Work out the finished part from the listing and answer in its coordinate system (mm). A direction names the side the tool comes from. Give positions to 0.01 mm unless a question says otherwise; leave off trailing zeros. Write each loop counter-clockwise with the first axis right and the second up, starting at its lowest first coordinate (ties: lowest second). Pieces come first, ordered by that corner, then holes. Notation, with made-up numbers: (85.25, 83.25) -> (136.25, 83.25) arc R22 ccw to (136.25, 109.25) -> close; hole circle Ø7 at (50, -21.75). An arc over 180 degrees is marked (long way). Use a Markdown table: item, result. Add a question column.
Q1. Section B-B, the plane z = -7.5 is taken. Give the vertices of the cut face in (x, y).
Q2. For faces 4 (the face through (-43, 10, -22.749)), 5 (the face through (-30.801, 10, -8)), 6 (the face through (-25, 9.25, 19)), 7 (the face through (-32, 14, 34.751)), determine the directions among +Z, -Z, +X, -X, +Y, -Y from which every point of the face is accessible in a straight line to the end or side of a thin tool.
Q3. Consider line 1 (X direction, y = 18.5, z = -2); line 2 (X direction, y = 7.5, z = -18); line 3 (X direction, y = 18.5, z = 15.5). Determine where each line is inside the solid, lowest interval first.
Q4. Section C-C, the plane x = -45 is taken. Give the vertices of the cut face in (y, z).
Q5. Section D-D, the plane z = 21 is taken. Give the vertices of the cut face in (x, y), plus the area to 3 significant figures.
Q6. For a pull along X with two mould halves and no side action, classify faces 1 (the face through (-26.999, 9.86, 9.807)), 2 (the face through (-51.47, 9.86, -29.92)), 3 (the face through (-25, 9.25, 41)) as pulls with the +X half, pulls with the -X half, needs draft (parallel to the pull), parting line crosses it, or undercut.
Q7. Section A-A, the plane y = 10 is taken. Give the vertices of the cut face in (x, z), plus the area to 3 significant figures.
Q8. Each of these flat-tipped pins is pushed along its axis until it touches: pin 1 Ø1 at (y, z) = (7, -4) entering from -X; pin 2 Ø1.6 at (x, y) = (-25, 10) entering from -Z; pin 3 Ø1.2 at (x, y) = (-27.5, 10) entering from -Z; pin 4 Ø2 at (x, z) = (-39.5, -7.5) entering from -Y. Where does it stop, or does it pass through?
from build123d import *

# Parameters (mm, degrees)
BOSS_EXTRUDE1_DEPTH = 20
SKETCH2_R           = 4
CUT_EXTRUDE2_DEPTH  = 8
SKETCH3_W           = 7.740011002
SKETCH3_H           = 1.5
SKETCH3_W_2         = 10.772479775
CUT_EXTRUDE4_DEPTH  = 10
SKETCH4_W           = 10
SKETCH4_H           = 15
CUT_EXTRUDE5_DEPTH  = 2


with BuildPart() as part:
    # Sketch1 → Boss-Extrude1 (new body)
    with BuildSketch(Plane(origin=(0, 0, 0), x_dir=(1, 0, 0), z_dir=(0, 1, 0))):
        with BuildLine():
            Line((-30.801242739, -7.293137555), (-30.801242739, 22.748893216))
            ThreePointArc((-30.801242739, 22.748893216), (-52.993630348, 31.941283464), (-43.801242739, 9.748894762))
            Line((-43.801242739, 9.748894762), (-43.801242739, -47.251105238))
            Line((-43.801242739, -47.251105238), (-41.301242739, -47.251105238))
            Line((-41.301242739, -47.251105238), (-41.301242739, 22.748894762))
            Line((-41.301242739, 22.748894762), (-43.801242739, 22.748894762))
            Line((-43.801242739, 22.748894762), (-43.801242739, 12.248894762))
            ThreePointArc((-43.801242739, 12.248894762), (-51.225863395, 30.173516511), (-33.301242739, 22.748893216))
            Line((-33.301242739, 22.748893216), (-33.301242739, -47.251106784))
            Line((-33.301242739, -47.251106784), (-23.301242739, -47.251106784))
            Line((-23.301242739, -47.251106784), (-23.301242739, -12.251106784))
            Line((-23.301242739, -12.251106784), (-30.801242739, -7.293137555))
        make_face()
    extrude(amount=BOSS_EXTRUDE1_DEPTH)

    # Sketch2 → Cut-Extrude2 (cut)
    with BuildSketch(Plane.ZY.offset(33.301242739)):
        with Locations((19.751105238, 10)):
            Circle(SKETCH2_R)
        with Locations((39.751105238, 10)):
            Circle(SKETCH2_R)
    extrude(amount=-CUT_EXTRUDE2_DEPTH, mode=Mode.SUBTRACT)

    # Sketch3 → Cut-Extrude4 (cut)
    with BuildSketch(Plane(origin=(-23.301242739, 0, 0), x_dir=(0, 0, -1), z_dir=(1, 0, 0))):
        with Locations((-40.137346671, 10)):
            Rectangle(SKETCH3_W, SKETCH3_H)
        with Locations((-29.751106784, 10)):
            Rectangle(SKETCH3_W_2, SKETCH3_H)
        with Locations((-19.364866896, 10)):
            Rectangle(SKETCH3_W, SKETCH3_H)
    extrude(amount=-CUT_EXTRUDE4_DEPTH, mode=Mode.SUBTRACT)

    # Sketch4 → Cut-Extrude5 (cut)
    with BuildSketch(Plane.ZY.offset(33.301242739)):
        with Locations((29.751105238, 10)):
            Rectangle(SKETCH4_W, SKETCH4_H)
    extrude(amount=-CUT_EXTRUDE5_DEPTH, mode=Mode.SUBTRACT)


solid = part.part
Result set:
| question | item | result |
|---|---|---|
| 1 | outline | (-43.8, 0) -> (-41.3, 0) -> (-41.3, 20) -> (-43.8, 20) -> close; (-33.3, 0) -> (-30.8, 0) -> (-30.8, 20) -> (-33.3, 20) -> close |
| 2 | face 4 | +Y, -Y |
| 2 | face 5 | -Z, +X, +Y, -Y |
| 2 | face 6 | +X |
| 2 | face 7 | none |
| 3 | line 1 | x = -43.8 to -41.3, -33.3 to -30.8 |
| 3 | line 2 | x = -55.9 to -53.17, -43.8 to -41.3, -33.3 to -30.8 |
| 3 | line 3 | x = -43.8 to -41.3, -33.3 to -23.3 |
| 4 | outline | (0, -35.69) -> (20, -35.69) -> (20, -33.18) -> (0, -33.18) -> close; (0, -12.32) -> (20, -12.32) -> (20, -9.8) -> (0, -9.8) -> close |
| 5 | outline | (-43.8, 0) -> (-41.3, 0) -> (-41.3, 20) -> (-43.8, 20) -> close; (-33.3, 0) -> (-23.3, 0) -> (-23.3, 9.25) -> (-25.3, 9.25) -> (-25.3, 6.2) -> (-33.3, 6.2) -> close; (-33.3, 13.8) -> (-25.3, 13.8) -> (-25.3, 10.75) -> (-23.3, 10.75) -> (-23.3, 20) -> (-33.3, 20) -> close |
| 5 | area | 186 mm2 |
| 6 | face 1 | pulls with the +X half |
| 6 | face 2 | undercut |
| 6 | face 3 | needs draft |
| 7 | outline | (-43.8, -22.75) -> (-41.3, -22.75) -> (-41.3, 47.25) -> (-43.8, 47.25) -> (-43.8, -9.75) arc R13 ccw (long way) to (-30.8, -22.75) -> (-30.8, 7.29) -> (-23.3, 12.25) -> (-23.3, 15.49) -> (-33.3, 15.49) -> (-33.3, -22.75) arc R10.5 cw (long way) to (-43.8, -12.25) -> close; (-33.3, 23.75) -> (-25.3, 23.75) -> (-25.3, 23.23) -> (-23.3, 23.23) -> (-23.3, 24.36) -> (-33.3, 24.36) -> close; (-33.3, 35.14) -> (-23.3, 35.14) -> (-23.3, 36.27) -> (-25.3, 36.27) -> (-25.3, 35.75) -> (-33.3, 35.75) -> close; (-33.3, 44.01) -> (-23.3, 44.01) -> (-23.3, 47.25) -> (-33.3, 47.25) -> close |
| 7 | area | 499 mm2 |
| 8 | pin 1 | stops at x = -43.8 |
| 8 | pin 2 | stops at z = 10.6 |
| 8 | pin 3 | stops at z = 9.08 |
| 8 | pin 4 | passes through |
